```python
from build123d import *

# Parameters (mm, degrees)
F0_R     = 7.5
F1_DEPTH = 25


with BuildPart() as f1:
    # F0 (on Front) → F1 (new body)
    with BuildSketch(Plane.XZ):
        with BuildLine():
            ThreePointArc((4.382898, -14.34539), (12.05702, -8.923467), (15, 0))
            ThreePointArc((15, 0), (-9.72197, 11.422929), (-2.397775, -14.807116))
            ThreePointArc((-2.397775, -14.807116), (1.019056, -14.965344), (4.382898, -14.34539))
        make_face()
        Circle(F0_R, mode=Mode.SUBTRACT)
        with BuildLine():
            ThreePointArc((4.382898, -14.34539), (1.019056, -14.965344), (-2.397775, -14.807116))
            Line((-2.397775, -14.807116), (-2.397775, -140.385768))
            ThreePointArc((-2.397775, -140.385768), (1.019056, -140.22754), (4.382898, -140.847494))
            Line((4.382898, -140.847494), (4.382898, -14.34539))
        make_face()
        with BuildLine():
            Line((-2.397775, -148.086501), (-2.397775, -140.385768))
            ThreePointArc((-2.397775, -140.385768), (-15, -155.192884), (-2.397775, -170))
            Line((-2.397775, -170), (-2.397775, -162.299267))
            ThreePointArc((-2.397775, -162.299267), (-7.5, -155.192884), (-2.397775, -148.086501))
        make_face()
        with BuildLine():
            ThreePointArc((4.382898, -140.847494), (1.019056, -140.22754), (-2.397775, -140.385768))
            Line((-2.397775, -140.385768), (-2.397775, -148.086501))
            ThreePointArc((-2.397775, -148.086501), (4.374168, -149.10054), (7.5, -155.192884))
            ThreePointArc((7.5, -155.192884), (4.374168, -161.285228), (-2.397775, -162.299267))
            Line((-2.397775, -162.299267), (-2.397775, -170))
            ThreePointArc((-2.397775, -170), (9.72197, -166.615813), (15, -155.192884))
            ThreePointArc((15, -155.192884), (12.05702, -146.269417), (4.382898, -140.847494))
        make_face()
    extrude(amount=F1_DEPTH)


solid = f1.part
```
Verification items for the finished model (mm, model axes). A direction names the side the tool comes from. Round coordinates to 2 decimals unless told otherwise and drop trailing zeros. Order: outer loops, then holes, each group sorted by start corner. A loop starts at its lowest first (then second) coordinate and runs counter-clockwise, first axis right, second up.
1) Material ranges on line 1 (Z direction, x = 0, y = -10); line 2 (Z direction, x = -1, y = -18.25); line 3 (Z direction, x = 6, y = -9.75), recorded low to high.
Geometry says:
line 1: z = -170.19 to -162.69, -147.69 to -7.5, 7.5 to 15
line 2: z = -170.16 to -162.63, -147.76 to -7.43, 7.43 to 14.97
line 3: z = -168.94 to -159.69, -150.69 to -141.45, -13.75 to -4.5, 4.5 to 13.75
2) Cross-section at B-B, the plane y = -3.75. Record the cut outline in (x, z).
Geometry says:
outline: (-2.4, -140.39) arc R15 ccw (long way) to (15, -155.19) arc R15 ccw to (4.38, -140.85) - (4.38, -14.35) arc R15 ccw to (15, 0) arc R15 ccw (long way) to (-2.4, -14.81) - close; hole circle Ø15 at (0, -155.19); hole circle Ø15 at (0, 0)
3) Cross-section at D-D, the plane z = -90. Record the cut outline in (x, y), plus the area to 3 significant figures.
Geometry says:
outline: (-2.4, -25) - (4.38, -25) - (4.38, 0) - (-2.4, 0) - close
area: 170 mm2
4) Cross-section at C-C, the plane x = 10. Record the cut outline in (y, z).
Geometry says:
outline: (-25, -166.37) - (0, -166.37) - (0, -144.01) - (-25, -144.01) - close; (-25, -11.18) - (0, -11.18) - (0, 11.18) - (-25, 11.18) - close
5) Cross-section at A-A, the plane x = 0. Record the cut outline in (y, z), plus the area to 3 significant figures.
Geometry says:
outline: (-25, -170.19) - (0, -170.19) - (0, -162.69) - (-25, -162.69) - close; (-25, -147.69) - (0, -147.69) - (0, -7.5) - (-25, -7.5) - close; (-25, 7.5) - (0, 7.5) - (0, 15) - (-25, 15) - close
area: 3,880 mm2
6) Tool access check on faces 1 (the flat face through (0, -25, -77)), 2 (the flat face through (-2.398, -12, -77)). Record the directions out of +Z, -Z, +X, -X, +Y, -Y that give a thin tool (end or side, any length) a straight path to the whole face; none if there is none.
Geometry says:
face 1: +Z, -Z, +X, -X, -Y
face 2: -X, +Y, -Y
7) Draft check along X on faces 3 (the flat face through (4.383, -12, -78)), 4 (the flat face through (0, 0, -77)), 5 (the cylindrical face through (-7.493, -12.325, 0.33)). Enter one of: +X half, -X half, draft (parallel to the pull), parting line (faces both ways), or undercut.
Geometry says:
face 3: +X half
face 4: draft
face 5: undercut
8) Depth check by flat-ended pin: pin 1 (1.5 mm diameter, centred on x = -12, y = -20.5, fed in from +Z); pin 2 (12.5 mm diameter, centred on y = -12.5, z = -92, fed in from +X); pin 3 (2 mm diameter, centred on y = -9, z = -93.5, fed in from -X). Enter the tip coordinate at first touch or a pass-through.
Geometry says:
pin 1: stops at z = 9.92
pin 2: stops at x = 4.38
pin 3: stops at x = -2.4
